from build123d import *

# Parameters (mm, degrees)
SKETCH1_25_W        = 26.4
SKETCH1_25_H        = 26.4
BOSS_EXTRUDE8_DEPTH = 20
SKETCH1_27_W        = 26.4
SKETCH1_27_H        = 26.4
BOSS_EXTRUDE9_DEPTH = 5
SKETCH1_R           = 10.5
CUT_EXTRUDE3_DEPTH  = 2
SKETCH4_R           = 1.4
CUT_EXTRUDE4_DEPTH  = 15


with BuildPart() as part:
    # Sketch1_25 → Boss-Extrude8 (new body)
    with BuildSketch(Plane.XY):
        Polygon((-46.914285714, 29.828571429), (-46.914285714, -1.887541502), (-46.914285714, -23.131847808), (-54.990816107, -70.171428571), (-35.990816107, -70.171428571), (-16.914285714, -24.770069728), (-16.914285714, -1.887541502), (-16.914285714, 29.828571429), align=None)
        with Locations((-31.914285714, 14.828571429)):
            Rectangle(SKETCH1_25_W, SKETCH1_25_H, mode=Mode.SUBTRACT)
    extrude(amount=-BOSS_EXTRUDE8_DEPTH)

    # Sketch1_27 → Boss-Extrude9 (add)
    with BuildSketch(Plane.XY):
        with Locations((-31.914285714, 14.828571429)):
            Rectangle(SKETCH1_27_W, SKETCH1_27_H)
        with BuildLine():
            Line((-28.605725915, 18.638938958), (-25.098574601, 22.146090272))
            ThreePointArc((-25.098574601, 22.146090272), (-31.889127352, 24.828539781), (-38.693091307, 22.180291958))
            Line((-38.693091307, 22.180291958), (-35.151738307, 18.638938958))
            ThreePointArc((-35.151738307, 18.638938958), (-36.914285714, 14.828571429), (-35.151738307, 11.018203899))
            Line((-35.151738307, 11.018203899), (-38.693091307, 7.4768509))
            ThreePointArc((-38.693091307, 7.4768509), (-31.867344715, 4.828681602), (-25.066760197, 7.540814964))
            Line((-25.066760197, 7.540814964), (-28.605725915, 11.079780683))
            ThreePointArc((-28.605725915, 11.079780683), (-26.916711196, 14.672850745), (-28.378751808, 18.364105335))
            Line((-28.378751808, 18.364105335), (-28.605725915, 18.638938958))
        make_face(mode=Mode.SUBTRACT)
    extrude(amount=-BOSS_EXTRUDE9_DEPTH)

    # Sketch1 → Cut-Extrude3 (cut)
    with BuildSketch(Plane.XY):
        with Locations((-31.914285714, 14.828571429)):
            Circle(SKETCH1_R)
    extrude(amount=-CUT_EXTRUDE3_DEPTH, mode=Mode.SUBTRACT)

    # Sketch4 → Cut-Extrude4 (cut)
    with BuildSketch(Plane(origin=(0, -70.171428571, 0), x_dir=(-1, 0, 0), z_dir=(0, -1, 0))):
        with Locations(Location((40.990816107, 12, 0), (0, 0, 90))):
            Circle(SKETCH4_R)
        with Locations(Location((49.990816107, 12, 0), (0, 0, 90))):
            Circle(SKETCH4_R)
    extrude(amount=-CUT_EXTRUDE4_DEPTH, mode=Mode.SUBTRACT)


solid = part.part
For this review, take the finished solid that the model builds, in its own axes (mm). A direction names the side the tool comes from. Round coordinates to 2 decimals unless told otherwise and drop trailing zeros. Loops run counter-clockwise (first coordinate to the right, second up) from the corner with the lowest first, then second, coordinate; pieces in that order, holes last. Notation, with made-up numbers: (44.5, 79.25) - (60.5, 79.25) arc R38 cw to (60.5, 117.25) - close; hole circle Ø2 at (35, -34.75). An arc over 180 degrees is marked (long way). One line per item, written item: value. Start each with the question number.
Item 1: For L1, parallel to X at y = 17, z = -9.25; L2, parallel to X at y = -58.75, z = -12; L3, parallel to X at y = -62.25, z = -12, list the stretches that pass through material, from the lowest coordinate up.
Item 2: Take a section at B-B (x = -44). Give the boundary of the cut face in (y, z).
Item 3: Clearance check with flat-ended pins moving along their axes: pin 1 Ø4 at (y, z) = (-50, -3.5) entering from +X; pin 2 Ø19 at (x, y) = (-31.91, 14.83) entering from +Z; pin 3 Ø0.8 at (x, z) = (-41, -12) entering from -Y. State where each tip first meets the part, or that it passes through.
Item 4: Take a section at D-D (y = -47.5). Give the boundary of the cut face in (x, z).
Item 5: For faces 1 (the cylindrical face through (-34.19, 4.58, -0.99)), 2 (the flat face through (-41, -55.171, -12)), 3 (the flat face through (-36.9, 9.27, -3.48)), list the 3-axis set-ups (+Z, -Z, +X, -X, +Y, -Y) from which the entire face can be reached by the end or side of a thin tool; tool diameter is ignored.
Item 6: Take a section at C-C (y = 13). Give the boundary of the cut face in (x, z), plus the area to 3 significant figures.
Item 7: The part is to be moulded in two halves that separate along Z. For faces 4 (the flat face through (-26.877, 20.368, -3.479)), 5 (the flat face through (-50, -55.171, -12)), 6 (the flat face through (-27, 13, -2)), 7 (the cylindrical face through (-51.36, -62.78, -11.7)), say which applies: +Z half, -Z half, draft (parallel to the pull), parting line (faces both ways), or undercut.
Item 8: Take a section at A-A (z = -12). Give the boundary of the cut face in (x, y), plus the area to 3 significant figures.
Answer below:
1. L1: x = -46.91 to -45.11, -18.71 to -16.91
1. L2: x = -53.03 to -51.39, -48.59 to -42.39, -39.59 to -31.19
1. L3: x = -53.63 to -51.39, -48.59 to -42.39, -39.59 to -32.66
2. outline: (-70.17, -20) - (1.63, -20) - (1.63, -5) - (28.03, -5) - (28.03, -20) - (29.83, -20) - (29.83, 0) - (-70.17, 0) - close
3. pin 1: stops at x = -26.67
3. pin 2: stops at z = -2
3. pin 3: stops at y = -55.17
4. outline: (-51.1, -20) - (-26.46, -20) - (-26.46, 0) - (-51.1, 0) - close
5. face 1: +Z
5. face 2: -Y
5. face 3: +Z, -Z
6. outline: (-46.91, -20) - (-45.11, -20) - (-45.11, -5) - (-36.57, -5) - (-36.57, -2) - (-42.25, -2) - (-42.25, 0) - (-46.91, 0) - close; (-27.26, -5) - (-18.71, -5) - (-18.71, -20) - (-16.91, -20) - (-16.91, 0) - (-21.57, 0) - (-21.57, -2) - (-27.26, -2) - close
6. area: 135 mm2
7. face 4: draft
7. face 5: undercut
7. face 6: +Z half
7. face 7: undercut
8. outline: (-54.99, -70.17) - (-51.39, -70.17) - (-51.39, -55.17) - (-48.59, -55.17) - (-48.59, -70.17) - (-42.39, -70.17) - (-42.39, -55.17) - (-39.59, -55.17) - (-39.59, -70.17) - (-35.99, -70.17) - (-16.91, -24.77) - (-16.91, 29.83) - (-46.91, 29.83) - (-46.91, -23.13) - close; hole (-45.11, 1.63) - (-18.71, 1.63) - (-18.71, 28.03) - (-45.11, 28.03) - close
8. area: 1,980 mm2
